Can you work these out from the model? Positions are in its coordinate system, mm. A direction names the side the tool comes from. Round coordinates to 2 decimals unless told otherwise and drop trailing zeros. Order: outer loops, then holes, each group sorted by start corner. A loop starts at its lowest first (then second) coordinate and runs counter-clockwise, first axis right, second up. Notation, with made-up numbers: M 5.5,86 L 32.5,86 A18 ccw 32.5,114 Z; hole C 22,74.5 d4. An arc over 180 degrees is marked long. Answer as a JSON object with one key per item and string values. Group by question number.
from build123d import *

# Parameters (mm, degrees)
F1_DEPTH = 1100
F2_R     = 8
F3_DEPTH = 3
F4_W     = 350
F4_H     = 90
F4_H_2   = 5
F5_DEPTH = 100.001
F7_START = -87
F6_W     = 90
F6_H     = 90
F6_R     = 6
F6_R_2   = 3
F7_DEPTH = 10
F8_W     = 90
F8_H     = 90
F8_R     = 6
F8_R_2   = 3
F9_DEPTH = 13


with BuildPart() as f1:
    # F0 (on Front) → F1 (new body)
    with BuildSketch(Plane.XZ):
        with BuildLine():
            ThreePointArc((50, 45), (48.5355339059, 48.5355339059), (45, 50))
            Line((45, 50), (-45, 50))
            ThreePointArc((-45, 50), (-48.5355339059, 48.5355339059), (-50, 45))
            Line((-50, 45), (-50, -45))
            ThreePointArc((-50, -45), (-48.5355339059, -48.5355339059), (-45, -50))
            Line((-45, -50), (45, -50))
            ThreePointArc((45, -50), (48.5355339059, -48.5355339059), (50, -45))
            Line((50, -45), (50, 45))
        make_face()
        with BuildLine():
            ThreePointArc((-47, 45), (-46.4142135624, 46.4142135624), (-45, 47))
            Line((-45, 47), (45, 47))
            ThreePointArc((45, 47), (46.4142135624, 46.4142135624), (47, 45))
            Line((47, 45), (47, -45))
            ThreePointArc((47, -45), (46.4142135624, -46.4142135624), (45, -47))
            Line((45, -47), (-45, -47))
            ThreePointArc((-45, -47), (-46.4142135624, -46.4142135624), (-47, -45))
            Line((-47, -45), (-47, 45))
        make_face(mode=Mode.SUBTRACT)
        with BuildLine():
            ThreePointArc((50, -55), (48.5355339059, -51.4644660941), (45, -50))
            Line((45, -50), (-45, -50))
            ThreePointArc((-45, -50), (-48.5355339059, -51.4644660941), (-50, -55))
            Line((-50, -55), (-50, -145))
            ThreePointArc((-50, -145), (-48.5355339059, -148.5355339059), (-45, -150))
            Line((-45, -150), (45, -150))
            ThreePointArc((45, -150), (48.5355339059, -148.5355339059), (50, -145))
            Line((50, -145), (50, -55))
        make_face()
        with BuildLine():
            ThreePointArc((-47, -55), (-46.4142135624, -53.5857864376), (-45, -53))
            Line((-45, -53), (45, -53))
            ThreePointArc((45, -53), (46.4142135624, -53.5857864376), (47, -55))
            Line((47, -55), (47, -145))
            ThreePointArc((47, -145), (46.4142135624, -146.4142135624), (45, -147))
            Line((45, -147), (-45, -147))
            ThreePointArc((-45, -147), (-46.4142135624, -146.4142135624), (-47, -145))
            Line((-47, -145), (-47, -55))
        make_face(mode=Mode.SUBTRACT)
    extrude(amount=-F1_DEPTH)

    # F2 (on face) → F3 (cut, through all)
    with BuildSketch(Plane.YZ.offset(50)):
        with Locations((170, 30)):
            Circle(F2_R)
    extrude(amount=-F3_DEPTH, mode=Mode.SUBTRACT)

    # F4 (on face) → F5 (cut, through all)
    with BuildSketch(Plane.YZ.offset(50)):
        with Locations((925, -100)):
            Rectangle(F4_W, F4_H)
        with Locations((925, -147.5)):
            Rectangle(F4_W, F4_H_2)
        with Locations((925, -52.5)):
            Rectangle(F4_W, F4_H_2)
    extrude(amount=-F5_DEPTH, mode=Mode.SUBTRACT)

    # F6 (on face) → F7 (join)
    with BuildSketch(Plane.YZ.offset(50).offset(F7_START)):
        with Locations((50, 0)):
            Rectangle(F6_W, F6_H)
        with Locations((21, -29)):
            Circle(F6_R, mode=Mode.SUBTRACT)
        with Locations((21, 29)):
            Circle(F6_R, mode=Mode.SUBTRACT)
        with Locations((79, -29)):
            Circle(F6_R, mode=Mode.SUBTRACT)
        with Locations((50, 0)):
            Circle(F6_R_2, mode=Mode.SUBTRACT)
        with Locations((79, 29)):
            Circle(F6_R, mode=Mode.SUBTRACT)
        with Locations((50, -100)):
            Rectangle(F6_W, F6_H)
        with Locations((21, -129)):
            Circle(F6_R, mode=Mode.SUBTRACT)
        with Locations((21, -71)):
            Circle(F6_R, mode=Mode.SUBTRACT)
        with Locations((50, -100)):
            Circle(F6_R_2, mode=Mode.SUBTRACT)
        with Locations((79, -129)):
            Circle(F6_R, mode=Mode.SUBTRACT)
        with Locations((79, -71)):
            Circle(F6_R, mode=Mode.SUBTRACT)
    extrude(amount=-F7_DEPTH)

    # F8 (on face) → F9 (join)
    with BuildSketch(Plane(origin=(0, 0, -50), x_dir=(1, 0, 0), z_dir=(0, 0, -1))):
        with Locations((0, -930)):
            Rectangle(F8_W, F8_H)
        with Locations((-29, -959)):
            Circle(F8_R, mode=Mode.SUBTRACT)
        with Locations((0, -930)):
            Circle(F8_R_2, mode=Mode.SUBTRACT)
        with Locations((29, -959)):
            Circle(F8_R, mode=Mode.SUBTRACT)
        with Locations((-29, -901)):
            Circle(F8_R, mode=Mode.SUBTRACT)
        with Locations((29, -901)):
            Circle(F8_R, mode=Mode.SUBTRACT)
    extrude(amount=-F9_DEPTH)


solid = f1.part
Item 1: Suppose I cut it at A-A, the plane z = -12. Write out the boundary of the cut face in (x, y).
Item 2: On a 3-axis mill with a long thin cutter (end or side, diameter ignored), from which of +Z, -Z, +X, -X, +Y, -Y can I reach the whole of each face in a straight line? I mean faces 4 (the face through (1, 1037, -47)), 5 (the face through (47, 542, 1)), 6 (the face through (1, 436, -47)). Say none if no direction works.
Item 3: Suppose I cut it at C-C, the plane y = 382. State how many separate pieces and enclosed holes the cut face has, and give its area (3 significant figures).
Item 4: I need wall thicknesses on line 1 (Z direction, x = 24, y = 705.5); line 2 (Y direction, x = 29, z = -41.75); line 3 (X direction, y = 901, z = -41.5). Which ranges of each line are inside material? Lowest first, please.
Item 5: Suppose I cut it at B-B, the plane x = -13.5. Write out the boundary of the cut face in (y, z).
Item 6: I'm going to push a flat-ended pin straight in: pin 1 Ø19 at (x, y) = (-29, 901) entering from -Z. Where does the tip first touch, or does it pass through?
Item 7: If we mould it in two halves opening along X, with no side actions, what happens to faces 1 (the face through (-50, 370, -99)), 2 (the face through (-4, 1100, -48)), 3 (the face through (-1, 939, -37))? For each: +X half, -X half, draft (parallel to the pull), parting line (faces both ways), or undercut.
Computed:
{
 "1": {"outline": "M -50,0 L -47,0 L -47,5 L -37,5 L -37,95 L -47,95 L -47,1100 L -50,1100 Z; M 47,0 L 50,0 L 50,1100 L 47,1100 Z"},
 "2": {"face 4": "+Y", "face 5": "+Y, -Y", "face 6": "-Y"},
 "3": {"separate pieces": "1", "enclosed holes": "2", "area": "2,290 mm^2"},
 "4": {"line 1": "z = -150 to -147, -53 to -47, 47 to 50", "line 2": "y = 885 to 895, 907 to 953, 965 to 975", "line 3": "x = -50 to -47, -45 to -35, -23 to 23, 35 to 45, 47 to 50"},
 "5": {"outline": "M 0,-150 L 750,-150 L 750,-147 L 0,-147 Z; M 0,-53 L 750,-53 L 750,-50 L 1100,-50 L 1100,-47 L 975,-47 L 975,-37 L 885,-37 L 885,-47 L 0,-47 Z; M 0,47 L 1100,47 L 1100,50 L 0,50 Z"},
 "6": {"pin 1": "stops at z = -50"},
 "7": {"face 1": "-X half", "face 2": "draft", "face 3": "undercut"}
}
